Input: part model. Units: mm. Frame: model coordinates. Face numbers are marked on the shaded views. A direction names the side the tool comes from. Give positions to 0.01 mm unless a question says otherwise; leave off trailing zeros. Loops run counter-clockwise (first coordinate to the right, second up) from the corner with the lowest first, then second, coordinate; pieces in that order, holes last.
from build123d import *

# Parameters (mm, degrees)
SKETCH1_W           = 30
SKETCH1_H           = 20
SKETCH1_W_2         = 2
SKETCH1_H_2         = 5
BOSS_EXTRUDE1_DEPTH = 2
SKETCH2_R           = 1.5
CUT_EXTRUDE1_DEPTH  = 10
SKETCH3_W           = 13
SKETCH3_H           = 20
CUT_EXTRUDE2_DEPTH  = 10


with BuildPart() as part:
    # Sketch1 → Boss-Extrude1 (new body)
    with BuildSketch(Plane(origin=(0, 0, 0), x_dir=(1, 0, 0), z_dir=(0, 1, 0))):
        Rectangle(SKETCH1_W, SKETCH1_H)
        with Locations((-1, 5)):
            Rectangle(SKETCH1_W_2, SKETCH1_H_2, mode=Mode.SUBTRACT)
        with Locations((-1, -5)):
            Rectangle(SKETCH1_W_2, SKETCH1_H_2, mode=Mode.SUBTRACT)
    extrude(amount=BOSS_EXTRUDE1_DEPTH)

    # Sketch2 → Cut-Extrude1 (cut)
    with BuildSketch(Plane(origin=(0, 2, 0), x_dir=(1, 0, 0), z_dir=(0, 1, 0))):
        with Locations(Location((-10, 5, 0), (0, 0, 270))):
            Circle(SKETCH2_R)
        with Locations(Location((-10, -5, 0), (0, 0, 270))):
            Circle(SKETCH2_R)
    extrude(amount=-CUT_EXTRUDE1_DEPTH, mode=Mode.SUBTRACT)

    # Sketch3 → Cut-Extrude2 (cut)
    with BuildSketch(Plane(origin=(0, 2, 0), x_dir=(1, 0, 0), z_dir=(0, 1, 0))):
        with Locations((-8.5, 0)):
            Rectangle(SKETCH3_W, SKETCH3_H)
    extrude(amount=-CUT_EXTRUDE2_DEPTH, mode=Mode.SUBTRACT)


solid = part.part
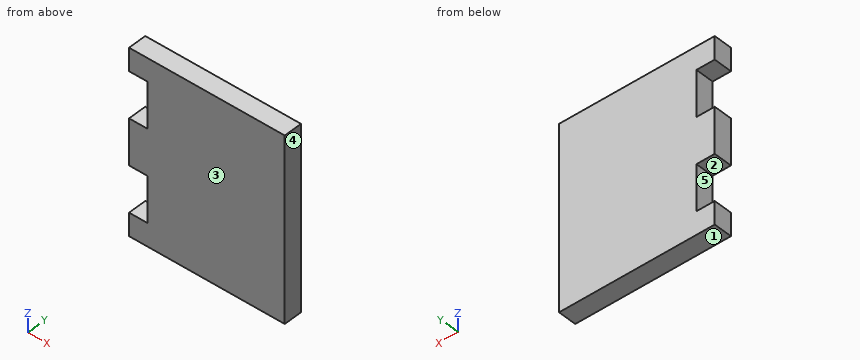
(1) Mould query, pull axis Z, two halves, no side actions, for the marked faces 1, 2 and 3. Classes: +Z half, -Z half, draft (parallel to the pull), parting line (faces both ways), or undercut.
Values follow:
face 1: -Z half
face 2: undercut
face 3: draft
(2) Pin query (flat end, axial travel): pin 1 Ø1 at (y, z) = (1, -5.5) entering from -X. Return the tip coordinate at first contact, or that it passes through.
Values follow:
pin 1: stops at x = 0
(3) Reachability of the marked faces 4 and 5 from +Z, -Z, +X, -X, +Y, -Y: full face, straight path, thin tool, end or side. Return the list, or none.
Values follow:
face 4: +Z, -Z, +X, +Y, -Y
face 5: -X, +Y, -Y
(4) Cut plane B-B (z = 4). Return the cut outline in (x, y).
Values follow:
outline: (0, 0) - (15, 0) - (15, 2) - (0, 2) - close
(5) Cut plane A-A (y = 0.95). Return the cut outline in (x, z), and give its area (3 significant figures).
Values follow:
outline: (-2, -10) - (15, -10) - (15, 10) - (-2, 10) - (-2, 7.5) - (0, 7.5) - (0, 2.5) - (-2, 2.5) - (-2, -2.5) - (0, -2.5) - (0, -7.5) - (-2, -7.5) - close
area: 320 mm2
(6) Ray query, probe 1 along X at (y, z) = (1.8, -5.5). Return the intervals inside material, ascending.
Values follow:
probe 1: x = 0 to 15
